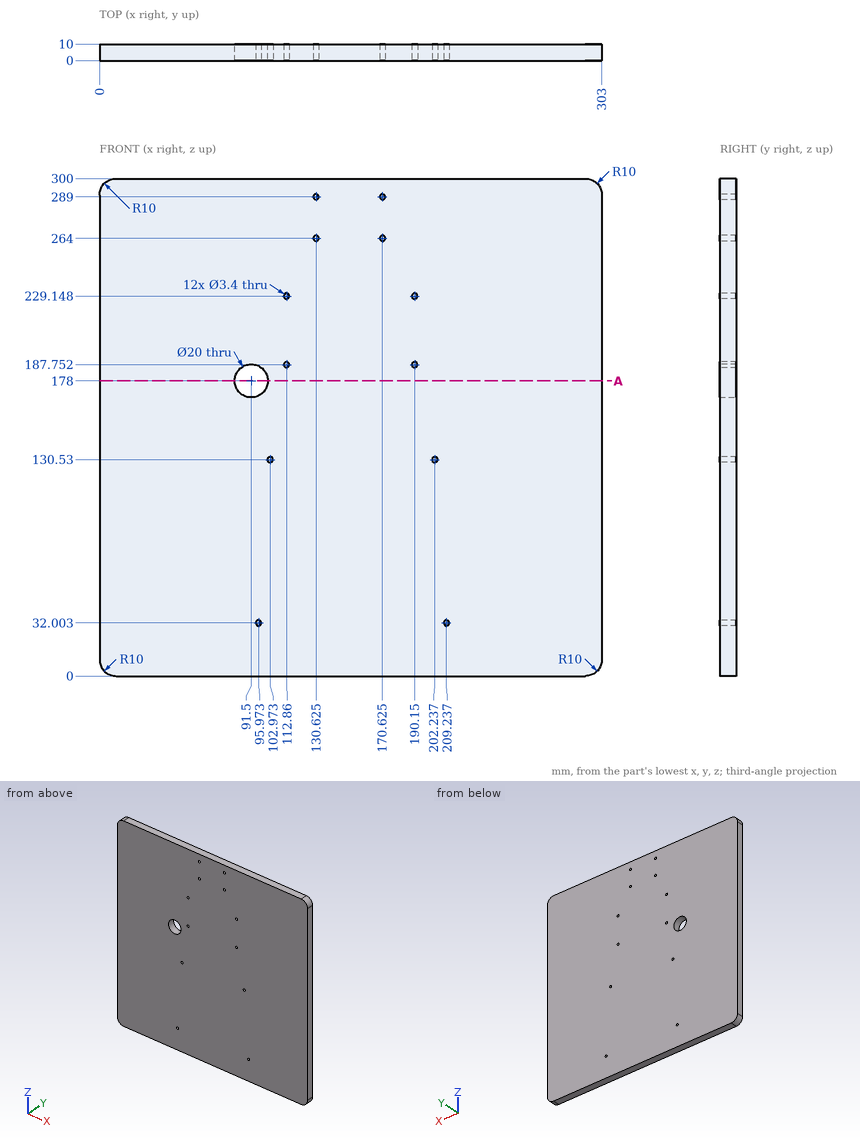
Could you check a few things on this drawing? It's one solid part, dimensions in mm from its lowest x, y, z. Coordinates: 2 decimals unless noted, no trailing zeros. Loops run counter-clockwise (first coordinate to the right, second up) from the corner with the lowest first, then second, coordinate; pieces in that order, holes last. Notation, with made-up numbers: (89.25, 42.5) - (131.25, 42.5) arc R20 ccw to (131.25, 46.5) - close; hole circle Ø2 at (32, -38.5). An arc over 180 degrees is marked (long way). Return JSON: item names as keys, results as strings. Group by question number.
Item 1: Will this pin go through, and if not, where does the flat tip stop? P1, Ø4.5, axis at x = 209.24, z = 32, coming from the -Y side.
Item 2: If we section it at A-A on z = 178: Write out the boundary of the cut face in (x, y).
Item 3: I need wall thicknesses on line 1 (X direction, y = 5.5, z = 264) (1 decimal); line 2 (Z direction, x = 112.86, y = 7); line 3 (Z direction, x = 190, y = 7) (1 decimal). Which ranges of each line are inside material? Lowest first, please. Write a range as from..to.
Calculated:
{
 "1": {"P1": "stops at y = 0"},
 "2": {"outline": "(0, 0) - (81.5, 0) - (81.5, 10) - (0, 10) - close; (101.5, 0) - (303, 0) - (303, 10) - (101.5, 10) - close"},
 "3": {"line 1": "x = 0..128.9, 132.3..168.9, 172.3..303", "line 2": "z = 0..186.05, 189.45..227.45, 230.85..300", "line 3": "z = 0..186.1, 189.4..227.5, 230.8..300"}
}
